Design review of the part built by this model. Coordinates are the model's own, in mm. A direction names the side the tool comes from. Give positions to 0.01 mm unless a question says otherwise; leave off trailing zeros. Order: outer loops, then holes, each group sorted by start corner. A loop starts at its lowest first (then second) coordinate and runs counter-clockwise, first axis right, second up. Notation, with made-up numbers: (41.25, 70.25) -> (67.25, 70.25) arc R23 cw to (67.25, 90.25) -> close; hole circle Ø10 at (80.5, -36). An arc over 180 degrees is marked (long way). Return JSON: item names as keys, results as strings.
Autodesk Inventor part; units mm, degrees
ref_plane "YZ Plane" through (0, 0, 0) normal (1, 0, 0) x (0, 1, 0)
ref_plane "XZ Plane" through (0, 0, 0) normal (0, 1, 0) x (-1, 0, 0)
ref_plane "XY Plane" through (0, 0, 0) normal (0, 0, 1) x (1, 0, 0)
sketch "Sketch1" plane through (0, 0, 0) normal (0, 1, 0) x (-1, 0, 0)
  line L0 (0, 0) -> (347, 0)
  line L1 (347, 0) -> (347, 60)
  line L2 (347, 60) -> (0, 60)
  line L3 (0, 60) -> (0, 0)
  dimension "d0" = 60
  dimension "d1" = 347
extrude "Extrusion1" add sketch "Sketch1" along normal blind 6
sketch "Sketch2" plane through (0, 6, 0) normal (0, 1, 0) x (1, 0, 0)
  line L0 (-347, 0) -> (-347, -60)
  line L1 (0, -60) -> (0, 0)
  line L2 (-347, -18) -> (-351, -18)
  line L3 (-353, -20) -> (-353, -24)
  line L4 (-351, -26) -> (-347, -26)
  line L5 (-347, -26) -> (-347, -18)
  line L6 (0, -18) -> (4, -18)
  line L7 (6, -20) -> (6, -24)
  line L8 (4, -26) -> (0, -26)
  line L9 (0, -26) -> (0, -18)
  arc A0 (-351, -18) -> (-353, -20) centre (-351, -20) ccw
  arc A1 (-353, -24) -> (-351, -26) centre (-351, -24) ccw
  arc A2 (6, -20) -> (4, -18) centre (4, -20) ccw
  arc A3 (4, -26) -> (6, -24) centre (4, -24) ccw
  line L10 (-347, -34) -> (-351, -34)
  line L11 (-353, -36) -> (-353, -40)
  line L12 (-351, -42) -> (-347, -42)
  line L13 (-347, -42) -> (-347, -34)
  line L14 (0, -34) -> (4, -34)
  line L15 (6, -36) -> (6, -40)
  line L16 (4, -42) -> (0, -42)
  line L17 (0, -42) -> (0, -34)
  arc A4 (-351, -34) -> (-353, -36) centre (-351, -36) ccw
  arc A5 (-353, -40) -> (-351, -42) centre (-351, -40) ccw
  arc A6 (6, -36) -> (4, -34) centre (4, -36) ccw
  arc A7 (4, -42) -> (6, -40) centre (4, -40) ccw
  line L18 (-349, -26) -> (-349, -34) construction
  point P0 (-349, -30)
  point P1 (-347, -30)
  dimension "d4" = 2
  dimension "d5" = 8
  dimension "d6" = 6
  dimension "d7" = 6
  dimension "d9" = 2
  dimension "d10" = 8
  dimension "d11" = 8
extrude "Extrusion2" add sketch "Sketch2" against normal blind 6
sketch "Sketch3" plane through (0, 6, 0) normal (0, 1, 0) x (1, 0, 0)
  line L0 (0, 0) -> (-347, 0)
  line L1 (-347, 0) -> (-347, -18)
  line L2 (-347, -60) -> (0, -60)
  line L3 (-330.7, -9.75) -> (-330.7, -14.25)
  line L4 (-347, -14.25) -> (-347, -9.75)
  line L5 (-342, -7.25) -> (-334.7, -7.25)
  line L6 (-334.7, -16.75) -> (-342, -16.75)
  line L7 (-347, -9.75) -> (-342, -9.75)
  line L8 (-334.7, -9.75) -> (-330.7, -9.75)
  line L9 (-330.7, -14.25) -> (-334.7, -14.25)
  line L10 (-342, -14.25) -> (-347, -14.25)
  line L11 (-342, -16.75) -> (-342, -14.25)
  line L12 (-342, -9.75) -> (-342, -7.25)
  line L13 (-334.7, -7.25) -> (-334.7, -9.75)
  line L14 (-334.7, -14.25) -> (-334.7, -16.75)
  line L15 (-330.7, -45.75) -> (-330.7, -50.25)
  line L16 (-347, -50.25) -> (-347, -45.75)
  line L17 (-342, -43.25) -> (-334.7, -43.25)
  line L18 (-334.7, -52.75) -> (-342, -52.75)
  line L19 (-347, -45.75) -> (-342, -45.75)
  line L20 (-334.7, -45.75) -> (-330.7, -45.75)
  line L21 (-330.7, -50.25) -> (-334.7, -50.25)
  line L22 (-342, -50.25) -> (-347, -50.25)
  line L23 (-342, -52.75) -> (-342, -50.25)
  line L24 (-342, -45.75) -> (-342, -43.25)
  line L25 (-334.7, -43.25) -> (-334.7, -45.75)
  line L26 (-334.7, -50.25) -> (-334.7, -52.75)
  line L27 (-173.5, -60) -> (-173.5, 0) construction
  line L28 (-16.3, -9.75) -> (-16.3, -14.25)
  line L29 (0, -14.25) -> (0, -9.75)
  line L30 (-5, -7.25) -> (-12.3, -7.25)
  line L31 (-12.3, -16.75) -> (-5, -16.75)
  line L32 (0, -9.75) -> (-5, -9.75)
  line L33 (-12.3, -9.75) -> (-16.3, -9.75)
  line L34 (-16.3, -14.25) -> (-12.3, -14.25)
  line L35 (-5, -14.25) -> (0, -14.25)
  line L36 (-5, -16.75) -> (-5, -14.25)
  line L37 (-5, -9.75) -> (-5, -7.25)
  line L38 (-12.3, -7.25) -> (-12.3, -9.75)
  line L39 (-12.3, -14.25) -> (-12.3, -16.75)
  line L40 (-16.3, -50.25) -> (-12.3, -50.25)
  line L41 (-16.3, -45.75) -> (-16.3, -50.25)
  line L42 (-12.3, -45.75) -> (-16.3, -45.75)
  line L43 (-12.3, -43.25) -> (-12.3, -45.75)
  line L44 (-12.3, -50.25) -> (-12.3, -52.75)
  line L45 (-5, -43.25) -> (-12.3, -43.25)
  line L46 (-12.3, -52.75) -> (-5, -52.75)
  line L47 (-5, -52.75) -> (-5, -50.25)
  line L48 (-5, -45.75) -> (-5, -43.25)
  line L49 (0, -45.75) -> (-5, -45.75)
  line L50 (-5, -50.25) -> (0, -50.25)
  line L51 (0, -50.25) -> (0, -45.75)
  point P0 (-347, -42)
  point P1 (-330.7, -12)
  point P2 (-330.7, -48)
  point P3 (-16.3, -12)
  point P4 (-16.3, -48)
  dimension "d14" = 4.5
  dimension "d15" = 2.5
  dimension "d16" = 2.5
  dimension "d17" = 5
  dimension "d18" = 4
  dimension "d19" = 7.3
  dimension "d20" = 4.5
  dimension "d21" = 2.5
  dimension "d22" = 2.5
  dimension "d23" = 5
  dimension "d24" = 4
  dimension "d25" = 7.3
  dimension "d26" = 6
  dimension "d27" = 6
extrude "Extrusion3" cut sketch "Sketch3" against normal blind 6
sketch "Sketch4" plane through (0, 6, 0) normal (0, 1, 0) x (1, 0, 0)
  line L0 (0, 0) -> (-347, 0)
  line L1 (-347, -60) -> (0, -60)
  line L2 (-5, -7.25) -> (-5, -9.75)
  line L3 (-322, 0) -> (-314, -8)
  line L4 (-314, -8) -> (-33, -8)
  line L5 (-33, -8) -> (-25, 0)
  line L6 (-322, -60) -> (-314, -52)
  line L7 (-314, -52) -> (-33, -52)
  line L8 (-33, -52) -> (-25, -60)
  dimension "d30" = 45
  dimension "d31" = 25
  dimension "d32" = 25
  dimension "d33" = 8
  dimension "d34" = 8
extrude "Extrusion4" cut sketch "Sketch4" against normal blind 6
equation "\"d16\" = d15"
equation "\"d22\" = d21"
equation "\"d34\" = d33"
properties part number "webcam_back_holder"
Item 1: Mouldability with a two-part tool opening along Z and no side actions: class faces 6 (the face through (0, 3, 30)), 7 (the face through (-318, 3, 56)), 8 (the face through (-29, 3, 4)), 9 (the face through (-338, 3, 16.75)) as released by +Z, released by -Z, zero draft, split by the parting line, or undercut.
Result set:
{"face 6": "undercut", "face 7": "released by +Z", "face 8": "released by -Z", "face 9": "undercut"}
Item 2: Wall thickness on L1, parallel to Z at x = -9, y = 2.5; L2, parallel to X at y = 4, z = 44; L3, parallel to X at y = 5.75, z = 40.5: over which ranges is each line inside the solid? List them lowest first. Write a range as [from, to].
Result set:
{"L1": "z = [0, 7.25], [16.75, 43.25], [52.75, 60]", "L2": "x = [-347, -342], [-334.7, -12.3], [-5, 0]", "L3": "x = [-352.94, 5.94]"}
Item 3: Add section A-A (x = -88.5). Give the boundary of the cut face in (y, z).
Result set:
{"outline": "(0, 8) -> (6, 8) -> (6, 52) -> (0, 52) -> close"}
Item 4: Machinability: for faces 1 (the face through (-29, 3, 56)), 2 (the face through (-347, 3, 5)), 3 (the face through (-347, 3, 30)), 4 (the face through (-9, 3, 43.25)), 5 (the face through (-175, 3, 8)), which of the approach directions +Z, -Z, +X, -X, +Y, -Y give a long, thin tool a straight path to every point of the face, cutting with its end or side? Answer none if there is none.
Result set:
{"face 1": "+Z, +Y, -Y", "face 2": "-Z, -X, +Y, -Y", "face 3": "-X, +Y, -Y", "face 4": "+Y, -Y", "face 5": "-Z, +Y, -Y"}
Item 5: For pin 1 (10 mm diameter, centred on x = -184, z = 22.5, fed in from -Y); pin 2 (1.2 mm diameter, centred on y = 2, z = 45, fed in from -X); pin 3 (3 mm diameter, centred on y = 3.5, z = 8, fed in from +X); pin 4 (2 mm diameter, centred on x = -269, y = 3, fed in from -Z), all flat-tipped, find the tip position at first contact; note any pin that passes through.
Result set:
{"pin 1": "stops at y = 0", "pin 2": "stops at x = -347", "pin 3": "stops at x = 0", "pin 4": "stops at z = 8"}
